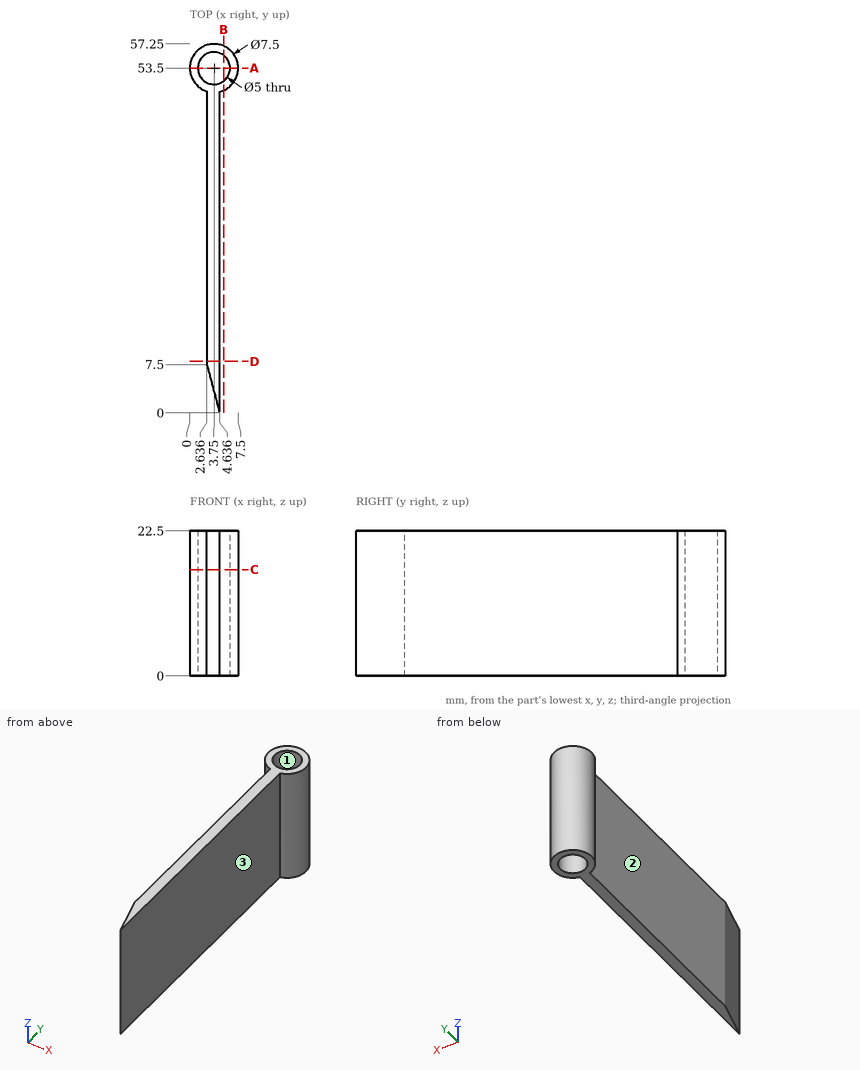
For this review, use the dimensioned drawing (mm, ordinates from the lowest corner) and the shaded views. Coordinates: 2 decimals unless noted, no trailing zeros. Write each loop counter-clockwise with the first axis right and the second up, starting at its lowest first coordinate (ties: lowest second). Pieces come first, ordered by that corner, then holes. Notation, with made-up numbers: (-38.5, 3.5) - (2.5, 3.5) arc R24 cw to (2.5, 27.5) - close; hole circle Ø2 at (-7.5, 67.25). An arc over 180 degrees is marked (long way). Answer in a Markdown table with one row per item. Add a question column.
Q1. Consider section A-A on y = 53.5. Give the boundary of the cut face in (x, z).
Q2. Clearance check with flat-ended pins moving along their axes: pin 1 (3 mm diameter, centred on y = 18, z = 19, fed in from +X); pin 2 (3 mm diameter, centred on y = 27.5, z = 14.5, fed in from -X). State where each tip first meets the part, or that it passes through.
Q3. Draft analysis for pull direction X (two halves, no side actions). For the marked faces 1, 2 and 3, state which applies: +X half, -X half, draft (parallel to the pull), parting line (faces both ways), or undercut.
Q4. Consider section D-D on y = 8. Give the boundary of the cut face in (x, z).
Q5. Consider section B-B on x = 5.25. Give the boundary of the cut face in (y, z).
Q6. To check wall thickness, follow line 1 along X through (y, z) = (10.5, 17.75); line 2 along Y through (x, z) = (2.25, 15.5) (1 decimal); line 3 along Y through (x, z) = (2, 21.25) (1 decimal). State the ranges of each line that lie inside material, in increasing order. Write a range as from..to.
Q7. Consider section C-C on z = 16.5. Give the boundary of the cut face in (x, y), then the cut area to 3 significant figures.
Answers below:
| question | item | result |
|---|---|---|
| 1 | outline | (0, 0) - (1.25, 0) - (1.25, 22.5) - (0, 22.5) - close; (6.25, 0) - (7.5, 0) - (7.5, 22.5) - (6.25, 22.5) - close |
| 2 | pin 1 | x = 4.64 |
| 2 | pin 2 | x = 2.64 |
| 3 | face 1 | undercut |
| 3 | face 2 | -X half |
| 3 | face 3 | +X half |
| 4 | outline | (2.64, 0) - (4.64, 0) - (4.64, 22.5) - (2.64, 22.5) - close |
| 5 | outline | (50.06, 0) - (51.5, 0) - (51.5, 22.5) - (50.06, 22.5) - close; (55.5, 0) - (56.94, 0) - (56.94, 22.5) - (55.5, 22.5) - close |
| 6 | line 1 | 2.64..4.64 |
| 6 | line 2 | 50.1..51.5, 55.5..56.9 |
| 6 | line 3 | 50.2..51.7, 55.3..56.8 |
| 7 | outline | (2.64, 7.5) - (4.64, 0) - (4.64, 49.86) arc R3.75 ccw (long way) to (2.64, 49.92) - close; hole circle Ø5 at (3.75, 53.5) |
| 7 | area | 117 mm² |
